```python
from build123d import *

# Parameters (mm, degrees)
SKETCH_1_W      = 125
SKETCH_1_H      = 19
EXTRUDE_1_DEPTH = 6
EXTRUDE_2_DEPTH = 50
SKETCH_3_W      = 125
SKETCH_3_H      = 19
EXTRUDE_3_DEPTH = 6


with BuildPart() as part:
    # 草图1 → 凸台-拉伸1 (new body)
    with BuildSketch(Plane.XY):
        Rectangle(SKETCH_1_W, SKETCH_1_H)
    extrude(amount=EXTRUDE_1_DEPTH)

    # 草图2 → 凸台-拉伸2 (add)
    with BuildSketch(Plane.XY.offset(6)):
        with BuildLine():
            Line((-62.5, 0), (-60.9, 0))
            ThreePointArc((-60.9, 0), (-53.9, -7), (-46.9, 0))
            Line((-46.9, 0), (-45.5, 0))
            ThreePointArc((-45.5, 0), (-38.5, -7), (-31.5, 0))
            Line((-31.5, 0), (-30.1, 0))
            ThreePointArc((-30.1, 0), (-23.1, -7), (-16.1, 0))
            Line((-16.1, 0), (-14.7, 0))
            ThreePointArc((-14.7, 0), (-7.7, -7), (-0.7, 0))
            Line((-0.7, 0), (0.7, 0))
            ThreePointArc((0.7, 0), (7.7, -7), (14.7, 0))
            Line((14.7, 0), (16.1, 0))
            ThreePointArc((16.1, 0), (23.1, -7), (30.1, 0))
            Line((30.1, 0), (31.5, 0))
            ThreePointArc((31.5, 0), (38.5, -7), (45.5, 0))
            Line((45.5, 0), (46.9, 0))
            ThreePointArc((46.9, 0), (53.9, -7), (60.9, 0))
            Line((60.9, 0), (62.5, 0))
            Line((62.5, 0), (62.5, -9.5))
            Line((62.5, -9.5), (-62.5, -9.5))
            Line((-62.5, -9.5), (-62.5, 0))
        make_face()
    extrude(amount=EXTRUDE_2_DEPTH)

    # 草图3 → 凸台-拉伸3 (add)
    with BuildSketch(Plane.XY.offset(56)):
        Rectangle(SKETCH_3_W, SKETCH_3_H)
    extrude(amount=EXTRUDE_3_DEPTH)


solid = part.part
```
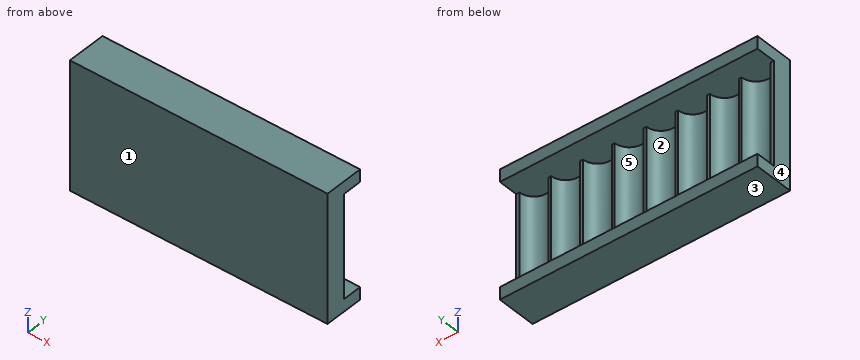
Could you check a few things on this model? Use its own coordinates, in mm. Face numbers are marked on the shaded views. A direction names the side the tool comes from. Coordinates: 2 decimals unless noted, no trailing zeros. Write each loop counter-clockwise with the first axis right and the second up, starting at its lowest first coordinate (ties: lowest second). Pieces come first, ordered by that corner, then holes. Notation, with made-up numbers: (6, 29) -> (29, 29) arc R17 ccw to (29, 44) -> close; hole circle Ø8 at (74, 45). An arc over 180 degrees is marked (long way). Write item = value, one per line. Start each with the question number.
(1) I want a section at C-C (z = 53). Please give me the cut outline in (x, y), plus the area to 3 significant figures.
(2) I want a section at B-B (x = 23.1). Please give me the cut outline in (y, z).
(3) I want a section at A-A (y = 7). Please give me the cut outline in (x, z).
(4) We'd pull the mould along Z, two halves only. Please class the marked faces 1, 2 and 3: released by +Z, released by -Z, zero draft, split by the parting line, or undercut.
(5) Which directions (+Z, -Z, +X, -X, +Y, -Y) give clear straight access to the entire face, cutting with the end or side of a thin tool? Please do the marked faces 4 and 5.
(6) Will these pins go through, and if not, where does the flat tip stop? pin 1 (0.8 mm diameter, centred on x = -62, z = 27, fed in from +Y); pin 2 (6 mm diameter, centred on x = -22, z = 43, fed in from +Y).
(7) I want a section at D-D (y = -2.5). Give the number of separate pieces and of enclosed holes in the cut face, plus the area to 3 significant figures.
(8) I need wall thicknesses on line 1 (Z direction, x = -51, y = 7.75); line 2 (Y direction, x = 55, z = 31.5); line 3 (Y direction, x = -53.5, z = 21.5). Which ranges of each line are inside material? Lowest first, please. Write a range as [from, to].
Result set:
q1.outline = (-62.5, -9.5) -> (62.5, -9.5) -> (62.5, 0) -> (60.9, 0) arc R7 cw to (46.9, 0) -> (45.5, 0) arc R7 cw to (31.5, 0) -> (30.1, 0) arc R7 cw to (16.1, 0) -> (14.7, 0) arc R7 cw to (0.7, 0) -> (-0.7, 0) arc R7 cw to (-14.7, 0) -> (-16.1, 0) arc R7 cw to (-30.1, 0) -> (-31.5, 0) arc R7 cw to (-45.5, 0) -> (-46.9, 0) arc R7 cw to (-60.9, 0) -> (-62.5, 0) -> close
q1.area = 572 mm2
q2.outline = (-9.5, 0) -> (9.5, 0) -> (9.5, 6) -> (-7, 6) -> (-7, 56) -> (9.5, 56) -> (9.5, 62) -> (-9.5, 62) -> close
q3.outline = (-62.5, 0) -> (62.5, 0) -> (62.5, 6) -> (-62.5, 6) -> close; (-62.5, 56) -> (62.5, 56) -> (62.5, 62) -> (-62.5, 62) -> close
q4.face_1 = zero draft
q4.face_2 = undercut
q4.face_3 = released by -Z
q5.face_4 = +Z, -Z, -X, +Y, -Y
q5.face_5 = +Y
q6.pin_1 = 0
q6.pin_2 = -5.67
q7.separate_pieces = 1
q7.enclosed_holes = 8
q7.area = 2,520 mm2
q8.line_1 = [0, 6], [56, 62]
q8.line_2 = [-9.5, -6.91]
q8.line_3 = [-9.5, -6.99]
